For this review, take the finished solid that the model builds, in its own axes (mm). Give positions to 0.01 mm unless a question says otherwise; leave off trailing zeros. Write each loop counter-clockwise with the first axis right and the second up, starting at its lowest first coordinate (ties: lowest second). Pieces come first, ordered by that corner, then holes. Notation, with made-up numbers: M -5.75,63.25 L 24.25,63.25 A30 cw 24.25,90.25 Z; hole C -12,48 d7. An arc over 180 degrees is marked long. One line per item, written item: value. Start each with the question number.
Item 1: Consider section A-A, the plane y = 1.1. Give the number of separate pieces and of enclosed holes in the cut face, and give its area (3 significant figures).
Item 2: Consider section B-B, the plane x = -69. Write out the cut boundary in (y, z), and give its area (3 significant figures).
Item 3: To check wall thickness, follow probe 1 along X at (y, z) = (4.75, -71); probe 2 along X at (y, z) = (1.1, -82); probe 3 along X at (y, z) = (0.95, -85.5). State the ranges of each line that lie inside material, in increasing order.
```python
from build123d import *

# Parameters (mm, degrees)
SKETCH1_W               = 6
SKETCH1_H               = 20
BOSS_EXTRUDE1_DEPTH     = 6
SKETCH2_W               = 6
SKETCH2_H               = 20
CUT_EXTRUDE1_DEPTH      = 179.986032975
CUT_EXTRUDE2_DEPTH      = 179.986032975
CUT_EXTRUDE2_DEPTH_BACK = 179.986032975
SKETCH3_W               = 10
SKETCH3_H               = 8
FILLET1_R               = 1


with BuildPart() as part:
    # Sketch1 → Boss-Extrude1 (new body)
    with BuildSketch(Plane(origin=(0, 0, 0), x_dir=(1, 0, 0), z_dir=(0, 1, 0))):
        with BuildLine():
            Line((-74, 0), (74, 0))
            ThreePointArc((74, 0), (78.242640687, 1.757359313), (80, 6))
            Line((80, 6), (80, 154))
            ThreePointArc((80, 154), (78.242640687, 158.242640687), (74, 160))
            Line((74, 160), (-74, 160))
            ThreePointArc((-74, 160), (-78.242640687, 158.242640687), (-80, 154))
            Line((-80, 154), (-80, 6))
            ThreePointArc((-80, 6), (-78.242640687, 1.757359313), (-74, 0))
        make_face()
        with Locations((-69, 80)):
            Rectangle(SKETCH1_W, SKETCH1_H, mode=Mode.SUBTRACT)
        with Locations((69, 80)):
            Rectangle(SKETCH1_W, SKETCH1_H, mode=Mode.SUBTRACT)
    extrude(amount=BOSS_EXTRUDE1_DEPTH)

    # Sketch2 → Cut-Extrude1 (cut, through all)
    with BuildSketch(Plane(origin=(0, 6, 0), x_dir=(1, 0, 0), z_dir=(0, 1, 0))):
        with Locations((23, 90)):
            Rectangle(SKETCH2_W, SKETCH2_H)
        with Locations((-23, 90)):
            Rectangle(SKETCH2_W, SKETCH2_H)
    extrude(amount=-CUT_EXTRUDE1_DEPTH, mode=Mode.SUBTRACT)

    # Sketch3 → Cut-Extrude2 (cut, two sides: drawn at the far end of the back side and taken through both)
    with BuildSketch(Plane(origin=(0, 6, 0), x_dir=(1, 0, 0), z_dir=(0, 1, 0)).offset(-CUT_EXTRUDE2_DEPTH_BACK)):
        with Locations((0, 80)):
            Rectangle(SKETCH3_W, SKETCH3_H)
    extrude(amount=CUT_EXTRUDE2_DEPTH + CUT_EXTRUDE2_DEPTH_BACK, mode=Mode.SUBTRACT)

    # Fillet1
    fillet1_edges = [part.edges().sort_by_distance(p)[0] for p in [
        (5, 3, -84),
        (5, 3, -76),
        (-5, 3, -76),
        (-5, 3, -84),
    ]]
    fillet(fillet1_edges, radius=FILLET1_R)


solid = part.part
```
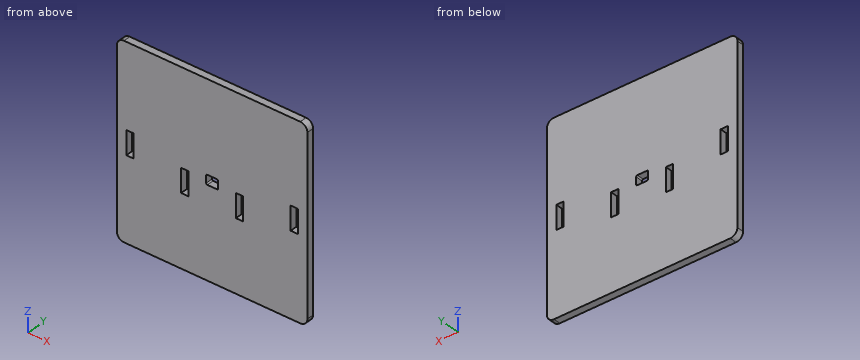
Model answer:
1. separate pieces: 1
1. enclosed holes: 5
1. area: 25,000 mm2
2. outline: M 0,-160 L 6,-160 L 6,-90 L 0,-90 Z; M 0,-70 L 6,-70 L 6,0 L 0,0 Z
2. area: 840 mm2
3. probe 1: x = -80 to -72, -66 to 66, 72 to 80
3. probe 2: x = -80 to -72, -66 to -26, -20 to -5, 5 to 20, 26 to 66, 72 to 80
3. probe 3: x = -80 to -72, -66 to -26, -20 to 20, 26 to 66, 72 to 80
